Could you check a few things on this model? Use its own coordinates, in mm. Coordinates: 2 decimals unless noted, no trailing zeros. Loops run counter-clockwise (first coordinate to the right, second up) from the corner with the lowest first, then second, coordinate; pieces in that order, holes last.
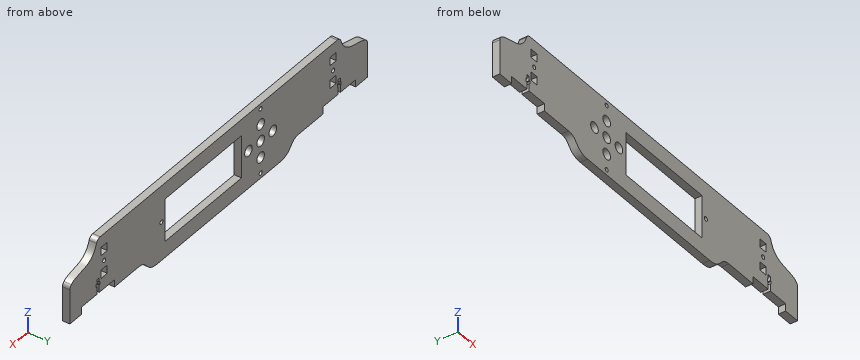
from build123d import *

# Parameters (mm, degrees)
F0_R     = 2
F0_W     = 8
F0_H     = 8
F0_R_2   = 5
F0_W_2   = 100
F0_H_2   = 41
F1_DEPTH = 7


with BuildPart() as f1:
    # F0 (on Front) → F1 (new body)
    with BuildSketch(Plane.XZ):
        with BuildLine():
            Line((-80, 0), (0, 0))
            Line((0, 0), (80, 0))
            add(Edge.make_bspline(
                [(80, 0), (96.28427, 0), (92.631489, 12.12483), (105, 12)],
                knots=[0, 0, 0, 0, 27.730849, 27.730849, 27.730849, 27.730849], degree=3))
            Line((105, 12), (136.5, 12))
            Line((136.5, 12), (136.5, 19))
            Line((136.5, 19), (156.5, 19))
            Line((156.5, 19), (156.5, 26))
            Line((156.5, 26), (155.5, 26))
            Line((155.5, 26), (155.5, 29))
            Line((155.5, 29), (156.5, 29))
            Line((156.5, 29), (156.5, 33.138553))
            Line((156.5, 33.138553), (158, 33.138553))
            Line((158, 33.138553), (159.5, 33.138553))
            Line((159.5, 33.138553), (159.5, 29))
            Line((159.5, 29), (160.5, 29))
            Line((160.5, 29), (160.5, 26))
            Line((160.5, 26), (159.5, 26))
            Line((159.5, 26), (159.5, 19))
            Line((159.5, 19), (179.5, 19))
            Line((179.5, 19), (179.5, 12))
            Line((179.5, 12), (195, 12))
            Line((195, 12), (195, 44.927057))
            ThreePointArc((195, 44.927057), (194.48614, 47.134895), (193.05018, 48.888925))
            add(Edge.make_bspline(
                [(160.114705, 68.542634), (166.272349, 49.558061), (183.983751, 55.869028), (193.05018, 48.888925)],
                knots=[2.170073, 2.170073, 2.170073, 2.170073, 40.679074, 40.679074, 40.679074, 40.679074], degree=3))
            ThreePointArc((160.114705, 68.542634), (158.298595, 71.044327), (155.358626, 72))
            Line((155.358626, 72), (0, 72))
            Line((0, 72), (-155.358626, 72))
            ThreePointArc((-155.358626, 72), (-158.298595, 71.044327), (-160.114705, 68.542634))
            add(Edge.make_bspline(
                [(-160.114705, 68.542634), (-166.272349, 49.558061), (-183.983751, 55.869028), (-193.05018, 48.888925)],
                knots=[2.170073, 2.170073, 2.170073, 2.170073, 40.679074, 40.679074, 40.679074, 40.679074], degree=3))
            ThreePointArc((-193.05018, 48.888925), (-194.48614, 47.134895), (-195, 44.927057))
            Line((-195, 44.927057), (-195, 12))
            Line((-195, 12), (-179.5, 12))
            Line((-179.5, 12), (-179.5, 19))
            Line((-179.5, 19), (-159.5, 19))
            Line((-159.5, 19), (-159.5, 26))
            Line((-159.5, 26), (-160.5, 26))
            Line((-160.5, 26), (-160.5, 29))
            Line((-160.5, 29), (-159.5, 29))
            Line((-159.5, 29), (-159.5, 33.138553))
            Line((-159.5, 33.138553), (-158, 33.138553))
            Line((-158, 33.138553), (-156.5, 33.138553))
            Line((-156.5, 33.138553), (-156.5, 29))
            Line((-156.5, 29), (-155.5, 29))
            Line((-155.5, 29), (-155.5, 26))
            Line((-155.5, 26), (-156.5, 26))
            Line((-156.5, 26), (-156.5, 19))
            Line((-156.5, 19), (-136.5, 19))
            Line((-136.5, 19), (-136.5, 12))
            Line((-136.5, 12), (-105, 12))
            add(Edge.make_bspline(
                [(-80, 0), (-96.28427, 0), (-92.631489, 12.12483), (-105, 12)],
                knots=[0, 0, 0, 0, 27.730849, 27.730849, 27.730849, 27.730849], degree=3))
        make_face()
        with Locations((-55, 5)):
            Circle(F0_R, mode=Mode.SUBTRACT)
        with Locations((-150, 35)):
            Rectangle(F0_W, F0_H, mode=Mode.SUBTRACT)
        with Locations((-55, 20)):
            Circle(F0_R_2, mode=Mode.SUBTRACT)
        with Locations((150, 35)):
            Rectangle(F0_W, F0_H, mode=Mode.SUBTRACT)
        with Locations((-150, 46)):
            Circle(F0_R, mode=Mode.SUBTRACT)
        with Locations((-71, 36)):
            Circle(F0_R_2, mode=Mode.SUBTRACT)
        with Locations((-55, 36)):
            Circle(F0_R_2, mode=Mode.SUBTRACT)
        with Locations((-39, 36)):
            Circle(F0_R_2, mode=Mode.SUBTRACT)
        with Locations((-55, 52)):
            Circle(F0_R_2, mode=Mode.SUBTRACT)
        with Locations((-150, 57)):
            Rectangle(F0_W, F0_H, mode=Mode.SUBTRACT)
        with Locations((-55, 67)):
            Circle(F0_R, mode=Mode.SUBTRACT)
        with Locations((20, 36)):
            Rectangle(F0_W_2, F0_H_2, mode=Mode.SUBTRACT)
        with Locations((75, 37)):
            Circle(F0_R, mode=Mode.SUBTRACT)
        with Locations((150, 46)):
            Circle(F0_R, mode=Mode.SUBTRACT)
        with Locations((150, 57)):
            Rectangle(F0_W, F0_H, mode=Mode.SUBTRACT)
    extrude(amount=F1_DEPTH)


solid = f1.part
(1) For pin 1 (0.5 mm diameter, centred on x = -160, y = -4.5, fed in from +Z); pin 2 (2.5 mm diameter, centred on x = 150, z = 46, fed in from -Y); pin 3 (2 mm diameter, centred on x = -165.5, y = -5, fed in from -Z); pin 4 (1 mm diameter, centred on y = -3, z = 49.5, fed in from +X), each with a flat end and sliding along its axis, tell me the tip position at first contact or that it passes through.
Answers:
pin 1: stops at z = 69.39
pin 2: passes through
pin 3: stops at z = 19
pin 4: stops at x = 192.9
(2) Imagine slicing it at A-A, the plane x = 38. Write out the boundary of the cut face in (y, z), and give its area (3 significant figures).
Answers:
outline: (-7, 0) - (0, 0) - (0, 15.5) - (-7, 15.5) - close; (-7, 56.5) - (0, 56.5) - (0, 72) - (-7, 72) - close
area: 217 mm2
(3) I need wall thicknesses on probe 1 along Z at (x, y) = (150, -3.75); probe 2 along Z at (x, y) = (-55, -1.5); probe 3 along Z at (x, y) = (-13, -5.25). Which ranges of each line are inside material? Lowest first, please.
Answers:
probe 1: z = 19 to 31, 39 to 44, 48 to 53, 61 to 72
probe 2: z = 0 to 3, 7 to 15, 25 to 31, 41 to 47, 57 to 65, 69 to 72
probe 3: z = 0 to 15.5, 56.5 to 72
(4) Imagine slicing it at C-C, the plane x = -109. Write out the boundary of the cut face in (y, z).
Answers:
outline: (-7, 12) - (0, 12) - (0, 72) - (-7, 72) - close
(5) Imagine slicing it at B-B, the plane y = -4.5. State how many separate pieces and enclosed holes the cut face has, and give its area (3 significant figures).
Answers:
separate pieces: 1
enclosed holes: 15
area: 18,900 mm2
